Verification items for this drawing (mm, ordinates from the low corner). A direction names the side the tool comes from. Round coordinates to 2 decimals unless told otherwise and drop trailing zeros. Order: outer loops, then holes, each group sorted by start corner. A loop starts at its lowest first (then second) coordinate and runs counter-clockwise, first axis right, second up. Notation, with made-up numbers: (54, -10.75) -> (106, -10.75) arc R24 ccw to (106, 24.25) -> close; hole circle Ø1 at (55.5, -28.75). An arc over 180 degrees is marked (long way). Put each result on its own line as item: value.
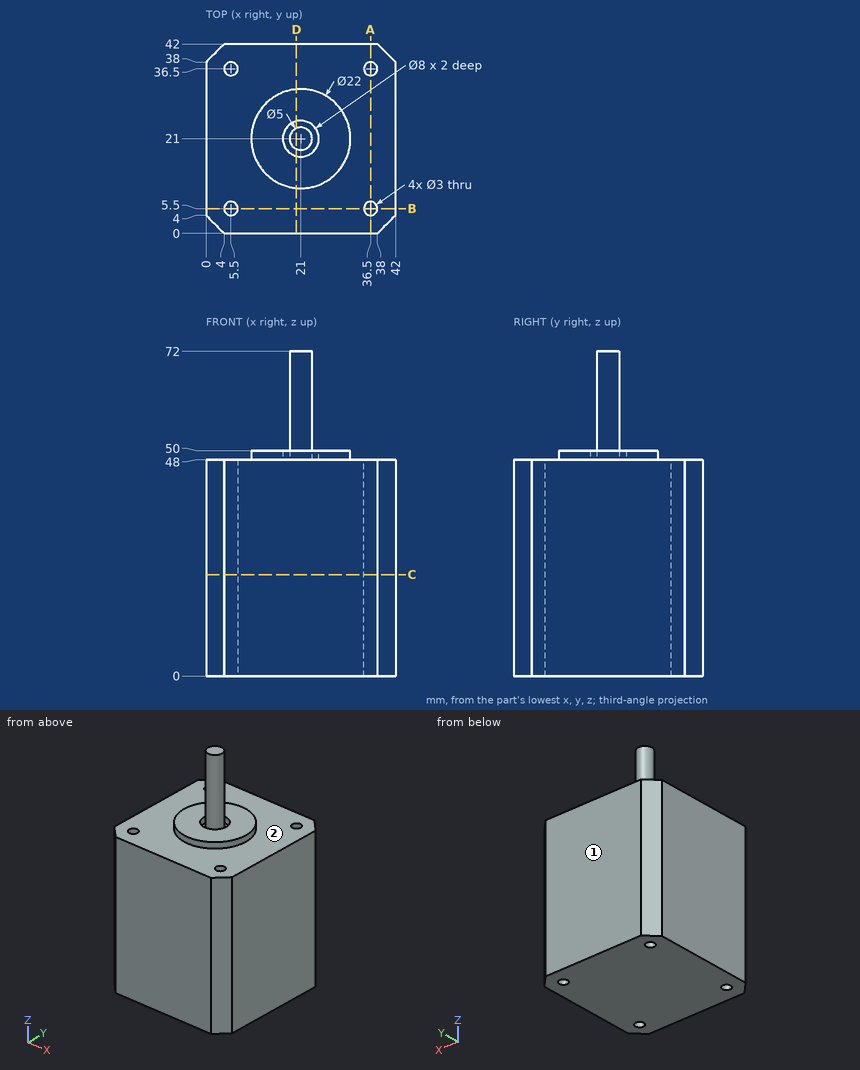
Item 1: Section check D-D on x = 20. Record the boundary of the cut face in (y, z), then the cut area to 3 significant figures.
Check sheet entries:
outline: (0, 0) -> (42, 0) -> (42, 48) -> (31.95, 48) -> (31.95, 50) -> (24.87, 50) -> (24.87, 48) -> (23.29, 48) -> (23.29, 72) -> (18.71, 72) -> (18.71, 48) -> (17.13, 48) -> (17.13, 50) -> (10.05, 50) -> (10.05, 48) -> (0, 48) -> close
area: 2,150 mm^2
Item 2: Tool access check on the marked faces 1 and 2. Record the directions out of +Z, -Z, +X, -X, +Y, -Y that give a thin tool (end or side, any length) a straight path to the whole face; none if there is none.
Check sheet entries:
face 1: +Z, -Z, +X, -X, +Y
face 2: +Z
Item 3: Gauge pin test, flat end, axial feed: pin 1 Ø4 at (x, y) = (5.5, 5.5) entering from +Z. Record the tip position at first contact, or that the pin passes through.
Check sheet entries:
pin 1: stops at z = 48
Item 4: Section check C-C on z = 22.5. Record the boundary of the cut face in (x, y), then the cut area to 3 significant figures.
Check sheet entries:
outline: (0, 4) -> (4, 0) -> (38, 0) -> (42, 4) -> (42, 38) -> (38, 42) -> (4, 42) -> (0, 38) -> close; hole circle Ø3 at (5.5, 5.5); hole circle Ø3 at (5.5, 36.5); hole circle Ø3 at (36.5, 5.5); hole circle Ø3 at (36.5, 36.5)
area: 1,700 mm^2
Item 5: Material ranges on L1, parallel to Y at x = 5.5, z = 19; L2, parallel to Y at x = 21, z = 48.75; L3, parallel to X at y = 36, z = 37, recorded low to high. Write a range as [from, to].
Check sheet entries:
L1: y = [0, 4], [7, 35], [38, 42]
L2: y = [10, 17], [18.5, 23.5], [25, 32]
L3: x = [0, 4.09], [6.91, 35.09], [37.91, 42]
Item 6: Section check A-A on x = 36.5. Record the boundary of the cut face in (y, z).
Check sheet entries:
outline: (0, 0) -> (4, 0) -> (4, 48) -> (0, 48) -> close; (7, 0) -> (35, 0) -> (35, 48) -> (7, 48) -> close; (38, 0) -> (42, 0) -> (42, 48) -> (38, 48) -> close
